```python
from build123d import *

# Parameters (mm, degrees)
F2_DEPTH      = 107
F2_DEPTH_BACK = 107
F0_R          = 18
F3_DEPTH      = 107
F3_DEPTH_BACK = 107
F1_R          = 18
F4_DEPTH      = 82
F4_DEPTH_BACK = 82


# Not quite as in the source:
# - a feature of the source that left no trace in its solid (it failed there, or was rolled back) is left out


with BuildPart() as f2:
    # F0 (on Front) → F2 (new body, two sides)
    with BuildSketch(Plane.XZ) as f2_sk:
        with BuildLine():
            ThreePointArc((-45.5, 20.1253140723), (-48, 20), (-50.5, 20.1253140723))
            Line((-50.5, 20.1253140723), (-50.5, -20.1253140723))
            ThreePointArc((-50.5, -20.1253140723), (-48, -20), (-45.5, -20.1253140723))
            Line((-45.5, -20.1253140723), (-45.5, 20.1253140723))
        make_face()
        with BuildLine():
            Line((-45.5, 20.1253140723), (-50.5, 20.1253140723))
            ThreePointArc((-50.5, 20.1253140723), (-48, 20), (-45.5, 20.1253140723))
        make_face()
        with BuildLine():
            ThreePointArc((-45.5, -20.1253140723), (-48, -20), (-50.5, -20.1253140723))
            Line((-50.5, -20.1253140723), (-45.5, -20.1253140723))
        make_face()
    extrude(amount=F2_DEPTH)
    extrude(f2_sk.sketch, amount=-F2_DEPTH_BACK)

    # F0 (on Front) → F3 (join, two sides)
    with BuildSketch(Plane.XZ) as f3_sk:
        with BuildLine():
            ThreePointArc((-45.5, 20.1253140723), (-29.4595037823, 28.2294901688), (-23, 45))
            ThreePointArc((-23, 45), (-64.7705098312, 63.5404962177), (-50.5, 20.1253140723))
            Line((-50.5, 20.1253140723), (-45.5, 20.1253140723))
        make_face()
        with Locations((-48, 45)):
            Circle(F0_R, mode=Mode.SUBTRACT)
        with BuildLine():
            Line((-45.5, -20.1253140723), (-50.5, -20.1253140723))
            ThreePointArc((-50.5, -20.1253140723), (-64.7705098312, -63.5404962177), (-23, -45))
            ThreePointArc((-23, -45), (-29.4595037823, -28.2294901688), (-45.5, -20.1253140723))
        make_face()
        with Locations((-48, -45)):
            Circle(F0_R, mode=Mode.SUBTRACT)
    extrude(amount=F3_DEPTH)
    extrude(f3_sk.sketch, amount=-F3_DEPTH_BACK)

    # F1 (on Top) → F4 (join, two sides)
    with BuildSketch(Plane.XY) as f4_sk:
        with BuildLine():
            ThreePointArc((2.5, 45.1253140723), (18.5404962177, 53.2294901688), (25, 70))
            ThreePointArc((25, 70), (-16.7705098312, 88.5404962177), (-2.5, 45.1253140723))
            Line((-2.5, 45.1253140723), (2.5, 45.1253140723))
        make_face()
        with Locations((0, 70)):
            Circle(F1_R, mode=Mode.SUBTRACT)
        with BuildLine():
            Line((2.5, 45.1253140723), (-2.5, 45.1253140723))
            ThreePointArc((-2.5, 45.1253140723), (0, 45), (2.5, 45.1253140723))
        make_face()
        with BuildLine():
            ThreePointArc((2.5, 45.1253140723), (0, 45), (-2.5, 45.1253140723))
            Line((-2.5, 45.1253140723), (-2.5, -45.1253140723))
            ThreePointArc((-2.5, -45.1253140723), (0, -45), (2.5, -45.1253140723))
            Line((2.5, -45.1253140723), (2.5, 45.1253140723))
        make_face()
        with BuildLine():
            ThreePointArc((2.5, -45.1253140723), (0, -45), (-2.5, -45.1253140723))
            Line((-2.5, -45.1253140723), (2.5, -45.1253140723))
        make_face()
        with BuildLine():
            Line((2.5, -45.1253140723), (-2.5, -45.1253140723))
            ThreePointArc((-2.5, -45.1253140723), (-16.7705098312, -88.5404962177), (25, -70))
            ThreePointArc((25, -70), (18.5404962177, -53.2294901688), (2.5, -45.1253140723))
        make_face()
        with Locations((0, -70)):
            Circle(F1_R, mode=Mode.SUBTRACT)
    extrude(amount=F4_DEPTH)
    extrude(f4_sk.sketch, amount=-F4_DEPTH_BACK)


solid = f2.part
```
Read the model definition and answer for the solid it produces. Units are mm, in the model's axes. A direction names the side the tool comes from. Give positions to 0.01 mm unless a question says otherwise; leave off trailing zeros. Loops run counter-clockwise (first coordinate to the right, second up) from the corner with the lowest first, then second, coordinate; pieces in that order, holes last.
Item 1: The part is cut by section C-C (x = -48). Write down the section's boundary in (y, z).
Item 2: For faces 4 (the flat face through (2.5, -1, 1)), 5 (the flat face through (-45.5, -1, 0)), 6 (the flat face through (-46, -107, 0)), determine the directions among +Z, -Z, +X, -X, +Y, -Y from which every point of the face is accessible in a straight line to the end or side of a thin tool.
Item 3: The part is cut by section A-A (y = -42). Write down the section's boundary in (x, z), and give its area (3 significant figures).
Item 4: Each of these flat-tipped pins is pushed along its axis until it touches: pin 1 Ø20 at (y, z) = (-18.5, -6) entering from -X; pin 2 Ø5 at (x, y) = (-29.5, 59) entering from -Z; pin 3 Ø2 at (y, z) = (75, -38) entering from -X; pin 4 Ø21.5 at (x, z) = (-48, 45) entering from +Y. Where does it stop, or does it pass through?
Item 5: The mould has two halves that part along X. Classify faces 1 (the flat face through (-50.5, -1, 0)), 2 (the flat face through (-2.5, 1, 1)), 3 (the flat face through (-2, -7, 82)): released by +X, released by -X, zero draft, split by the parting line, or undercut.
Item 6: The part is cut by section D-D (z = -45). Write down the section's boundary in (x, y).
Item 7: Find the intervals of material crossed by line 1 along Y through (x, z) = (0, 62); line 2 along X through (y, z) = (-54, -48); line 3 along Z through (x, y) = (-48, -46), in increasing order.
Item 8: The part is cut by section B-B (z = -7). Write down the section's boundary in (x, y).
Taken from the geometry:
1. outline: (-107, -70) - (107, -70) - (107, -63) - (-107, -63) - close; (-107, -27) - (107, -27) - (107, 27) - (-107, 27) - close; (-107, 63) - (107, 63) - (107, 70) - (-107, 70) - close
2. face 4: +Z, -Z, +X
2. face 5: +Y, -Y
2. face 6: +Z, -Z, +X, -X, -Y
3. outline: (-50.5, -20.13) arc R25 ccw (long way) to (-45.5, -20.13) - (-45.5, 20.13) arc R25 ccw (long way) to (-50.5, 20.13) - close; (-2.5, -82) - (2.5, -82) - (2.5, 82) - (-2.5, 82) - close; hole circle Ø36 at (-48, -45); hole circle Ø36 at (-48, 45)
3. area: 2,910 mm2
4. pin 1: stops at x = -50.5
4. pin 2: stops at z = -64.21
4. pin 3: stops at x = -72.27
4. pin 4: passes through
5. face 1: released by -X
5. face 2: undercut
5. face 3: zero draft
6. outline: (-73, -107) - (-66, -107) - (-66, 107) - (-73, 107) - close; (-30, -107) - (-23, -107) - (-23, -79.8) arc R25 ccw (long way) to (2.5, -45.13) - (2.5, 45.13) arc R25 ccw (long way) to (-23, 79.8) - (-23, 107) - (-30, 107) - close; hole (-23, -60.2) arc R25 cw to (-2.5, -45.13) - (-2.5, 45.13) arc R25 cw to (-23, 60.2) - close; hole circle Ø36 at (0, -70); hole circle Ø36 at (0, 70)
7. line 1: y = -95 to -88, -52 to 52, 88 to 95
7. line 2: x = -72.82 to -65.75, -30.25 to -23.18, -19.21 to -8.25, 8.25 to 19.21
7. line 3: z = -70 to -63, -27 to 27, 63 to 70
8. outline: (-50.5, -107) - (-45.5, -107) - (-45.5, 107) - (-50.5, 107) - close; (-2.5, -45.13) arc R25 ccw (long way) to (2.5, -45.13) - (2.5, 45.13) arc R25 ccw (long way) to (-2.5, 45.13) - close; hole circle Ø36 at (0, -70); hole circle Ø36 at (0, 70)
